Autodesk Fusion 360 part; units mm, degrees
sketch "Sketch2" plane through (0, 0, 0) normal (0, 0, 1) x (1, 0, 0)
  line L0 (-1.5076, -2.2009) -> (1.5076, -2.2009)
  line L1 (-1.5744, 2.1537) -> (1.5744, 2.1537)
  arc A0 (1.5076, -2.2009) -> (1.5744, 2.1537) centre (0, 0) ccw
  arc A1 (-1.5744, 2.1537) -> (-1.5076, -2.2009) centre (0, 0) ccw
  circle A2 centre (-1.9, 0.1) radius 0.3
  circle A3 centre (1.65, 0.1) radius 0.3
  dimension "d3" = 0.6
  dimension "d4" = 0.6
extrude "Extrude1" add sketch "Sketch2" along normal blind 2.1 contours L0 L1 A0 A1 | A2 | A3
extrude "Extrude2" add sketch "Sketch2" along normal blind 6 from surface at 2.1 contours A2 | A3
Design review of the part built by this model. Coordinates are the model's own, in mm. Round coordinates to 2 decimals unless told otherwise and drop trailing zeros. Write each loop counter-clockwise with the first axis right and the second up, starting at its lowest first coordinate (ties: lowest second). Pieces come first, ordered by that corner, then holes. Notation, with made-up numbers: M -34,-14.75 L 14,-14.75 A6 cw 14,-4.75 Z; hole C -30.5,-15.5 d10. An arc over 180 degrees is marked long. One line per item, written item: value. Start each with the question number.
1. Clearance check with flat-ended pins moving along their axes: P1, Ø2, axis at x = 0, y = -0.5, coming from the +Z side; P2, Ø2, axis at y = 1, z = 3, coming from the +X side; P3, Ø2, axis at x = -2, z = 4.5, coming from the +Y side. State where each tip first meets the part, or that it passes through.
2. Take a section at C-C on y = 0.1. State the section outline as (x, z) points, then the cut area to 3 significant figures.
3. Take a section at A-A on z = 5.5. State the section outline as (x, y) points, then the cut area to 3 significant figures.
4. Take a section at B-B on x = -1.7. State the section outline as (y, z) points.
5. Take a section at D-D on z = 2. State the section outline as (x, y) points.
6. To check wall thickness, follow probe 1 along Z at (x, y) = (-2.4, 0.2); probe 2 along X at (y, z) = (0.9, 1.5); probe 3 along Y at (x, z) = (-2.1, 7.75). State the ranges of each line that lie inside material, in increasing order. Write a range as from..to.
Computed:
1. P1: stops at z = 2.1
1. P2: stops at x = 2.61
1. P3: stops at y = 0.4
2. outline: M -2.67,0 L 2.67,0 L 2.67,2.1 L 1.95,2.1 L 1.95,8.1 L 1.35,8.1 L 1.35,2.1 L -1.6,2.1 L -1.6,8.1 L -2.2,8.1 L -2.2,2.1 L -2.67,2.1 Z
2. area: 18.4 mm²
3. outline: C -1.9,0.1 d0.6; C 1.65,0.1 d0.6
3. area: 0.565 mm²
4. outline: M -2.06,0 L 2.06,0 L 2.06,2.1 L 0.32,2.1 L 0.32,8.1 L -0.12,8.1 L -0.12,2.1 L -2.06,2.1 Z
5. outline: M -1.57,2.15 A2.67 ccw -1.51,-2.2 L 1.51,-2.2 A2.67 ccw 1.57,2.15 Z
6. probe 1: z = 0..2.1
6. probe 2: x = -2.51..2.51
6. probe 3: y = -0.12..0.32
